Part model, mm, in its own coordinate system. Round coordinates to 2 decimals unless told otherwise and drop trailing zeros. Order: outer loops, then holes, each group sorted by start corner. A loop starts at its lowest first (then second) coordinate and runs counter-clockwise, first axis right, second up. Notation, with made-up numbers: (-36.75, 30.5) - (-16.75, 30.5) arc R28 cw to (-16.75, 69.5) - close; hole circle Ø11 at (-29.75, 27). An arc over 180 degrees is marked (long way). Return JSON: item names as keys, results as strings. Group by question number.
Item 1: Saw through at A-A on z = 0.6. List the corners of the cut face in (x, y), and give its area (3 significant figures).
Item 2: Drop flat-ended pins along their axis: pin 1 (1 mm diameter, centred on y = 87, z = 1, fed in from +X); pin 2 (1 mm diameter, centred on x = 854.5, z = 1, fed in from +Y). Give the stop position or say it passes through.
Item 3: Probe probe 1 along Y at (x, z) = (809.5, 0.15); probe 2 along X at (y, z) = (79, 0.5); probe 3 along X at (y, z) = (66.5, 1.2). List the from-to ranges inside material, lowest first.
Item 4: Saw through at B-B on x = 754. List the corners of the cut face in (y, z).
```python
from build123d import *

# Parameters (mm, degrees)
BOSS_EXTRU_1_DEPTH = 2
CONG_1_R           = 20


with BuildPart() as part:
    # Esquisse1 → Boss.-Extru.1 (new body)
    with BuildSketch(Plane.XY):
        Polygon((653.5, 120), (669.5, 120), (669.5, 60), (969.5, 60), (969.5, 0), (653.5, 0), (-653.5, 0), (-653.5, 120), align=None)
    extrude(amount=BOSS_EXTRU_1_DEPTH)

    # Congé1
    cong_1_edges = [part.edges().sort_by_distance(p)[0] for p in [
        (669.5, 120, 1),
        (669.5, 60, 1),
        (969.5, 60, 1),
    ]]
    fillet(cong_1_edges, radius=CONG_1_R)


solid = part.part
```
Filled in:
{
 "1": {"outline": "(-653.5, 0) - (969.5, 0) - (969.5, 40) arc R20 ccw to (949.5, 60) - (689.5, 60) arc R20 cw to (669.5, 80) - (669.5, 100) arc R20 ccw to (649.5, 120) - (-653.5, 120) - close", "area": "177,000 mm^2"},
 "2": {"pin 1": "stops at x = 669.5", "pin 2": "stops at y = 60"},
 "3": {"probe 1": "y = 0 to 60", "probe 2": "x = -653.5 to 669.53", "probe 3": "x = -653.5 to 674.74"},
 "4": {"outline": "(0, 0) - (60, 0) - (60, 2) - (0, 2) - close"}
}
